The listing builds one solid part. Answer for the finished solid, in the listing's coordinates (mm). Round coordinates to 2 decimals unless told otherwise and drop trailing zeros. Order: outer loops, then holes, each group sorted by start corner. A loop starts at its lowest first (then second) coordinate and runs counter-clockwise, first axis right, second up. Notation, with made-up numbers: (-3, 1) -> (16, 1) arc R20 cw to (16, 15) -> close; hole circle Ø3 at (21.5, 66). An arc over 180 degrees is marked (long way). Return JSON: item names as keys, results as strings. Group by question number.
(1) The part is cut by section B-B (y = 2.5). Count the separate pieces of the cut face and the enclosed holes in it, plus the area to 3 significant figures.
(2) Consider line 1 (X direction, y = 3.25, z = 0) (3 decimals); line 2 (X direction, y = 3.3, z = 15); line 3 (X direction, y = 2.7, z = 27.05) (3 decimals). Determine where each line is inside the solid, lowest interval first. Write a range as [from, to].
(3) Each of these flat-tipped pins is pushed along its axis until it touches: pin 1 (3 mm diameter, centred on x = -21.88, z = 15.9, fed in from -Y); pin 2 (2 mm diameter, centred on y = 3.5, z = 10.5, fed in from -X). Where does it stop, or does it pass through?
(4) The part is cut by section A-A (z = 0). Determine the outline of the cut face in (x, y) (3 decimals), plus the area to 4 significant figures.
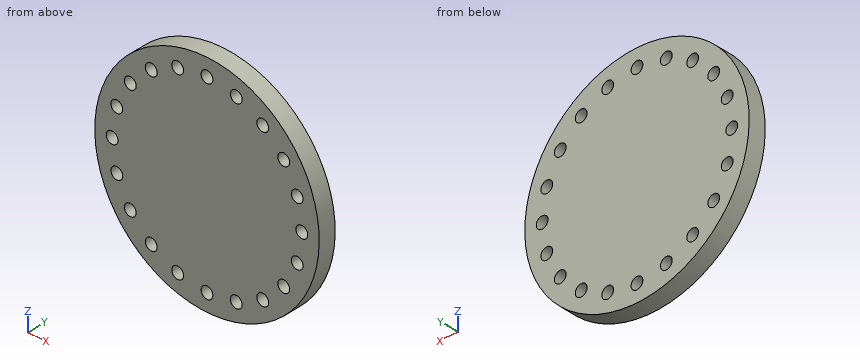
from build123d import *

# Parameters (mm, degrees)
SKETCH1_R           = 32
SKETCH1_R_2         = 1.675
BOSS_EXTRUDE1_DEPTH = 5


with BuildPart() as part:
    # Sketch1 → Boss-Extrude1 (new body)
    with BuildSketch(Plane(origin=(0, 0, 0), x_dir=(1, 0, 0), z_dir=(0, 1, 0))):
        with Locations(Location((0, 0, 0), (0, 0, 270))):
            Circle(SKETCH1_R)
        with Locations(Location((0, -27.05, 0), (0, 0, 270))):
            Circle(SKETCH1_R_2, mode=Mode.SUBTRACT)
        with Locations(Location((-8.358909698, -25.726078766, 0), (0, 0, 270))):
            Circle(SKETCH1_R_2, mode=Mode.SUBTRACT)
        with Locations(Location((-15.899591075, -21.883909698, 0), (0, 0, 270))):
            Circle(SKETCH1_R_2, mode=Mode.SUBTRACT)
        with Locations(Location((-21.883909698, -15.899591075, 0), (0, 0, 270))):
            Circle(SKETCH1_R_2, mode=Mode.SUBTRACT)
        with Locations(Location((-25.726078766, -8.358909698, 0), (0, 0, 270))):
            Circle(SKETCH1_R_2, mode=Mode.SUBTRACT)
        with Locations(Location((-27.05, 0, 0), (0, 0, 270))):
            Circle(SKETCH1_R_2, mode=Mode.SUBTRACT)
        with Locations(Location((-25.726078766, 8.358909698, 0), (0, 0, 270))):
            Circle(SKETCH1_R_2, mode=Mode.SUBTRACT)
        with Locations(Location((-21.883909698, 15.899591075, 0), (0, 0, 270))):
            Circle(SKETCH1_R_2, mode=Mode.SUBTRACT)
        with Locations(Location((-15.899591075, 21.883909698, 0), (0, 0, 270))):
            Circle(SKETCH1_R_2, mode=Mode.SUBTRACT)
        with Locations(Location((-8.358909698, 25.726078766, 0), (0, 0, 270))):
            Circle(SKETCH1_R_2, mode=Mode.SUBTRACT)
        with Locations(Location((0, 27.05, 0), (0, 0, 270))):
            Circle(SKETCH1_R_2, mode=Mode.SUBTRACT)
        with Locations(Location((8.358909698, 25.726078766, 0), (0, 0, 270))):
            Circle(SKETCH1_R_2, mode=Mode.SUBTRACT)
        with Locations(Location((15.899591075, 21.883909698, 0), (0, 0, 270))):
            Circle(SKETCH1_R_2, mode=Mode.SUBTRACT)
        with Locations(Location((21.883909698, 15.899591075, 0), (0, 0, 270))):
            Circle(SKETCH1_R_2, mode=Mode.SUBTRACT)
        with Locations(Location((25.726078766, 8.358909698, 0), (0, 0, 270))):
            Circle(SKETCH1_R_2, mode=Mode.SUBTRACT)
        with Locations(Location((27.05, 0, 0), (0, 0, 270))):
            Circle(SKETCH1_R_2, mode=Mode.SUBTRACT)
        with Locations(Location((25.726078766, -8.358909698, 0), (0, 0, 270))):
            Circle(SKETCH1_R_2, mode=Mode.SUBTRACT)
        with Locations(Location((21.883909698, -15.899591075, 0), (0, 0, 270))):
            Circle(SKETCH1_R_2, mode=Mode.SUBTRACT)
        with Locations(Location((15.899591075, -21.883909698, 0), (0, 0, 270))):
            Circle(SKETCH1_R_2, mode=Mode.SUBTRACT)
        with Locations(Location((8.358909698, -25.726078766, 0), (0, 0, 270))):
            Circle(SKETCH1_R_2, mode=Mode.SUBTRACT)
    extrude(amount=BOSS_EXTRUDE1_DEPTH)


solid = part.part
Answer below:
{
 "1": {"separate pieces": "1", "enclosed holes": "20", "area": "3,040 mm²"},
 "2": {"line 1": "x = [-32, -28.725], [-25.375, 25.375], [28.725, 32]", "line 2": "x = [-28.27, -23.3], [-20.47, 20.47], [23.3, 28.27]", "line 3": "x = [-17.097, -9.385], [-7.333, -1.675], [1.675, 7.333], [9.385, 17.097]"},
 "3": {"pin 1": "passes through", "pin 2": "stops at x = -30.56"},
 "4": {"outline": "(-32, 0) -> (-28.725, 0) -> (-28.725, 5) -> (-32, 5) -> close; (-25.375, 0) -> (25.375, 0) -> (25.375, 5) -> (-25.375, 5) -> close; (28.725, 0) -> (32, 0) -> (32, 5) -> (28.725, 5) -> close", "area": "286.5 mm²"}
}
